Check sheet for the drawn part. Datum: minimum x, y, z corner. Units: mm. Coordinates: 2 decimals unless noted, no trailing zeros. Order: outer loops, then holes, each group sorted by start corner. A loop starts at its lowest first (then second) coordinate and runs counter-clockwise, first axis right, second up. Notation, with made-up numbers: (16, -27) - (37, -27) arc R11 ccw to (37, -15) - close; hole circle Ø4 at (6.5, -22). An arc over 180 degrees is marked (long way). Put each result on its own line as item: value.
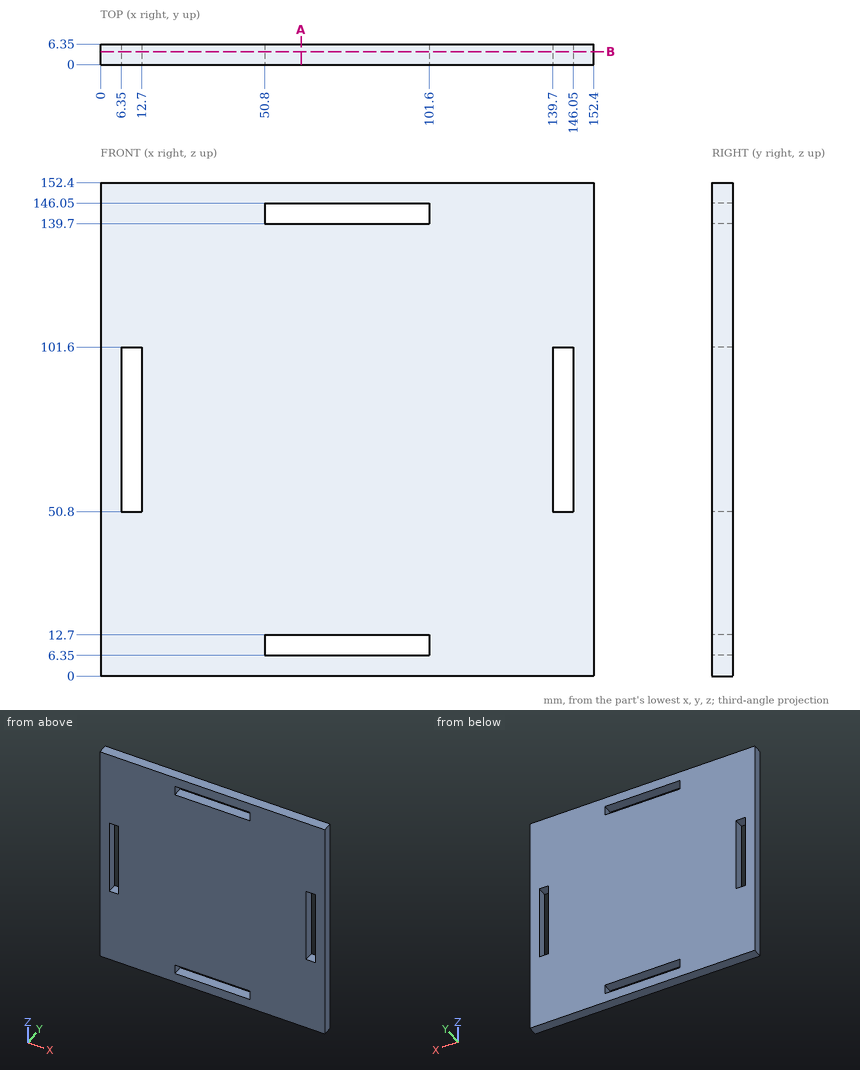
Q1. Depth check by flat-ended pin: pin 1 Ø3 at (x, y) = (73.5, 2.5) entering from -Z. Enter the tip coordinate at first touch or a pass-through.
Answer block:
pin 1: stops at z = 0
Q2. Section check A-A on x = 62. Record the boundary of the cut face in (y, z), then the cut area to 3 significant figures.
Answer block:
outline: (0, 0) - (6.35, 0) - (6.35, 6.35) - (0, 6.35) - close; (0, 12.7) - (6.35, 12.7) - (6.35, 139.7) - (0, 139.7) - close; (0, 146.05) - (6.35, 146.05) - (6.35, 152.4) - (0, 152.4) - close
area: 887 mm^2
Q3. Section check B-B on y = 4. Record the boundary of the cut face in (x, z).
Answer block:
outline: (0, 0) - (152.4, 0) - (152.4, 152.4) - (0, 152.4) - close; hole (6.35, 50.8) - (12.7, 50.8) - (12.7, 101.6) - (6.35, 101.6) - close; hole (50.8, 6.35) - (101.6, 6.35) - (101.6, 12.7) - (50.8, 12.7) - close; hole (50.8, 139.7) - (101.6, 139.7) - (101.6, 146.05) - (50.8, 146.05) - close; hole (139.7, 50.8) - (146.05, 50.8) - (146.05, 101.6) - (139.7, 101.6) - close
Q4. Thickness scan on L1, parallel to Z at x = 87, y = 1; L2, parallel to X at y = 1.25, z = 10. Record the ranges inside material, lowest first. Write a range as [from, to].
Answer block:
L1: z = [0, 6.35], [12.7, 139.7], [146.05, 152.4]
L2: x = [0, 50.8], [101.6, 152.4]
